Check sheet for the modelled part. Datum: model origin and axes. Units: mm. A direction names the side the tool comes from. Coordinates: 2 decimals unless noted, no trailing zeros. Loops run counter-clockwise (first coordinate to the right, second up) from the corner with the lowest first, then second, coordinate; pieces in that order, holes last.
```python
from build123d import *

# Parameters (mm, degrees)
SKETCH_R           = 7
PAD_DEPTH          = 61
SKETCH001_R        = 5.425
POCKET_DEPTH       = 61.001
POCKET001_DEPTH    = 5
SKETCH004_W        = 4
SKETCH004_H        = 10
POCKET002_DEPTH    = 5
POLARPATTERN_COUNT = 5


with BuildPart() as part:
    # Sketch → Pad (new body)
    with BuildSketch(Plane.XY):
        Circle(SKETCH_R)
    extrude(amount=PAD_DEPTH)

    # Sketch001 (on Face3 of Pad) → Pocket (cut, through all)
    with BuildSketch(Plane.XY.offset(61)):
        Circle(SKETCH001_R)
    extrude(amount=-POCKET_DEPTH, mode=Mode.SUBTRACT)

    # Sketch002 (on DatumPlane) → Groove (revolve, cut)
    with BuildSketch(Plane(origin=(0, 0, 30.5), x_dir=(0, 0, -1), z_dir=(1, 0, 0))):
        Polygon((9.5, 6), (11.25, 9.031089), (7.75, 9.031089), align=None)
        Polygon((-8.25, 9.031089), (-11.75, 9.031089), (-10, 6), align=None)
    revolve(axis=Axis((0, 0, 0), (0, 0, 1)), mode=Mode.SUBTRACT)

    # Sketch003 (on DatumPlane) → Pocket001 (cut)
    with BuildSketch(Plane.YZ.offset(7)):
        Polygon((0, 4.732051), (-1.5, 2.133975), (1.5, 2.133975), align=None)
    extrude(amount=-POCKET001_DEPTH, mode=Mode.SUBTRACT)

    # Sketch004 (on DatumPlane) → Pocket002 (cut)
    with BuildSketch(Plane.YZ.offset(7)):
        with Locations((0, 40.5)):
            Rectangle(SKETCH004_W, SKETCH004_H)
        with Locations((0, 21)):
            Rectangle(SKETCH004_W, SKETCH004_H)
    pocket002 = extrude(amount=-POCKET002_DEPTH, mode=Mode.SUBTRACT)

    # PolarPattern: Pocket002 ×5 about axis
    polarpattern_axis = Axis((0, 0, 0), (0, 0, 1))
    for i in range(1, POLARPATTERN_COUNT):
        add(pocket002.rotate(polarpattern_axis, i * 360 / POLARPATTERN_COUNT), mode=Mode.SUBTRACT)


solid = part.part
```
1) Section check A-A on x = 1.75. Enter the section's corners in (y, z) (3 decimals), plus the area to 3 significant figures.
Answer sheet:
outline: (-6.778, 0) - (-5.135, 0) - (-5.135, 16) - (-6.778, 16) - close; (-6.778, 26) - (-5.135, 26) - (-5.135, 35.5) - (-6.778, 35.5) - close; (-6.778, 45.5) - (-5.135, 45.5) - (-5.135, 61) - (-6.778, 61) - close; (5.135, 0) - (6.778, 0) - (6.778, 16) - (5.135, 16) - close; (5.135, 26) - (6.778, 26) - (6.778, 35.5) - (5.135, 35.5) - close; (5.135, 45.5) - (6.778, 45.5) - (6.778, 61) - (5.135, 61) - close
area: 135 mm2
2) Mould release check, pull along Y, two halves, no side actions. Record for faces 1 (the flat face through (6, 0, 35.5)), 2 (the cylindrical face through (6.466, -2.681, 30.622)): +Y half, -Y half, draft (parallel to the pull), parting line (faces both ways), or undercut.
Answer sheet:
face 1: undercut
face 2: parting line
3) Depth check by flat-ended pin: pin 1 (1.8 mm diameter, centred on x = 6, z = 19, fed in from +Y); pin 2 (1 mm diameter, centred on y = -5, z = 54.5, fed in from -X); pin 3 (1 mm diameter, centred on y = 4, z = 33.5, fed in from -X). Enter the tip coordinate at first touch or a pass-through.
Answer sheet:
pin 1: stops at y = 4.79
pin 2: stops at x = -5.36
pin 3: stops at x = -6.06
4) Scan lines: line 1 (Z direction, x = 2.75, y = 5); line 2 (Y direction, x = 0, z = 46) (3 decimals); line 3 (X direction, y = -5, z = 50). Record each from-to range of solid material in increasing order.
Answer sheet:
line 1: z = 0 to 16, 26 to 35.5, 45.5 to 61
line 2: y = -7 to -5.425, 5.425 to 7
line 3: x = -4.9 to -2.1, 2.1 to 4.9
5) Set-up check for faces 3 (the flat face through (5.5, 2, 20.9)), 4 (the flat face through (-3.138, -4.752, 40.43)), 5 (the flat face through (-5, -4, 26)), 6 (the cylindrical face through (-4.305, -3.301, 30.927)): record each of +Z, -Z, +X, -X, +Y, -Y from which the full face is reachable in a straight line by a thin tool's end or side.
Answer sheet:
face 3: +X
face 4: -X
face 5: none
face 6: +Z, -Z
